Source: CAD feature listing. Evaluate the final solid. Frame: model axes, mm. Give positions to 0.01 mm unless a question says otherwise; leave off trailing zeros. Write each loop counter-clockwise with the first axis right and the second up, starting at its lowest first coordinate (ties: lowest second). Pieces come first, ordered by that corner, then holes. Notation, with made-up numbers: (78, 0) -> (90, 0) arc R28 ccw to (90, 30) -> close; hole circle Ø10 at (31, -36). An arc over 180 degrees is marked (long way). Write item = value, one per line.
from build123d import *

# Parameters (mm, degrees)
EXTRUDE_1_4_DEPTH = 3.175
SKETCH4_R         = 2
M4_DRILL_DEPTH    = 8
SKETCH5_R         = 2
M4_DRILL2_DEPTH   = 8
SKETCH6_R         = 2.25
M4_THROUGH_DEPTH  = 6.35
SKETCH8_R         = 2.25
M4_THROUGH2_DEPTH = 10


with BuildPart() as part:
    # Sketch1 → 1/4 (new, symmetric)
    with BuildSketch(Plane.XY):
        Polygon((-20, 45), (20, 45), (30, 10), (30, -45), (-30, -45), (-30, 10), align=None)
    extrude(amount=EXTRUDE_1_4_DEPTH, both=True)

    # Sketch4 → M4_DRILL (cut)
    with BuildSketch(Plane(origin=(0, 45, 0), x_dir=(1, 0, 0), z_dir=(0, 1, 0))):
        with Locations(Location((-12, 0, 0), (0, 0, 180))):
            Circle(SKETCH4_R)
        with Locations((12, 0)):
            Circle(SKETCH4_R)
    extrude(amount=-M4_DRILL_DEPTH, mode=Mode.SUBTRACT)

    # Sketch5 → M4_DRILL2 (cut)
    with BuildSketch(Plane(origin=(0, -45, 0), x_dir=(-1, 0, 0), z_dir=(0, -1, 0))):
        with Locations(Location((-20, 0, 0), (0, 0, 180))):
            Circle(SKETCH5_R)
        with Locations((20, 0)):
            Circle(SKETCH5_R)
        with Locations(Location((0, 0, 0), (0, 0, 180))):
            Circle(SKETCH5_R)
    extrude(amount=-M4_DRILL2_DEPTH, mode=Mode.SUBTRACT)

    # Sketch6 → M4_through (cut)
    with BuildSketch(Plane.XY.offset(3.175)):
        with Locations((-25.2375, -31)):
            Circle(SKETCH6_R)
        with Locations((25.2375, -31)):
            Circle(SKETCH6_R)
        with Locations((-15.2375, 31)):
            Circle(SKETCH6_R)
        with Locations((15.2375, 31)):
            Circle(SKETCH6_R)
    extrude(amount=-M4_THROUGH_DEPTH, mode=Mode.SUBTRACT)

    # Sketch8 → M4_through2 (cut)
    with BuildSketch(Plane(origin=(0, 0, -3.175), x_dir=(-1, 0, 0), z_dir=(0, 0, -1))):
        with Locations((0, 16.5)):
            Circle(SKETCH8_R)
        with Locations((16.5, 0)):
            Circle(SKETCH8_R)
        with Locations((0, -16.5)):
            Circle(SKETCH8_R)
        with Locations((-16.5, 0)):
            Circle(SKETCH8_R)
    extrude(amount=-M4_THROUGH2_DEPTH, mode=Mode.SUBTRACT)


solid = part.part
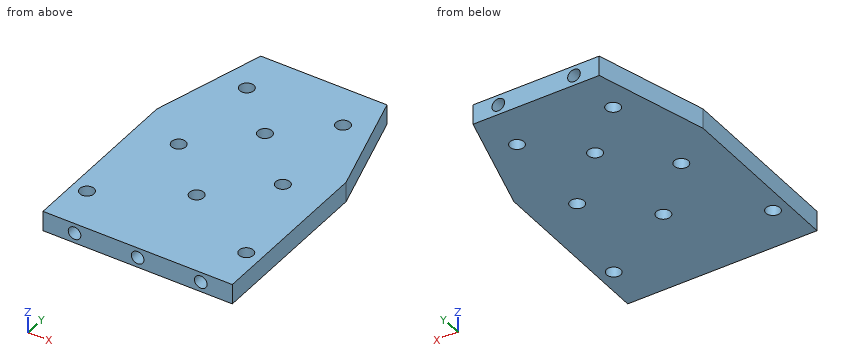
1) Material intervals for L1, parallel to Y at x = -16, z = 0.75; L2, parallel to X at y = -1.5, z = -1.75; L3, parallel to Y at x = -0.5, z = 1, sorted ascending.
Computed:
L1 = -45 to -2.19, 2.19 to 28.88, 33.12 to 45
L2 = -30 to -18.18, -14.82 to 14.82, 18.18 to 30
L3 = -37 to -18.69, -14.31 to 14.31, 18.69 to 45
2) Cut plane A-A (y = -16.5). Return the cut outline in (x, z) (3 decimals), then the cut area to 3 significant figures.
Computed:
outline = (-30, -3.175) -> (-2.25, -3.175) -> (-2.25, 3.175) -> (-30, 3.175) -> close; (2.25, -3.175) -> (30, -3.175) -> (30, 3.175) -> (2.25, 3.175) -> close
area = 352 mm²
3) Cut plane D-D (y = -32). Return the cut outline in (x, z) (3 decimals), then the cut area to 3 significant figures.
Computed:
outline = (-30, -3.175) -> (-27.253, -3.175) -> (-27.253, 3.175) -> (-30, 3.175) -> close; (-23.222, -3.175) -> (23.222, -3.175) -> (23.222, 3.175) -> (-23.222, 3.175) -> close; (27.253, -3.175) -> (30, -3.175) -> (30, 3.175) -> (27.253, 3.175) -> close
area = 330 mm²
4) Cut plane B-B (x = 0). Return the cut outline in (y, z) (3 decimals).
Computed:
outline = (-45, -3.175) -> (-18.75, -3.175) -> (-18.75, 3.175) -> (-45, 3.175) -> (-45, 2) -> (-37, 2) -> (-37, -2) -> (-45, -2) -> close; (-14.25, -3.175) -> (14.25, -3.175) -> (14.25, 3.175) -> (-14.25, 3.175) -> close; (18.75, -3.175) -> (45, -3.175) -> (45, 3.175) -> (18.75, 3.175) -> close
5) Contact query for flat-ended pins moving along their axis: pin 1 (3.5 mm diameter, centred on x = 0, z = 0, fed in from -Y); pin 2 (3 mm diameter, centred on x = 12, z = 0, fed in from +Y). Output: stop coordinate, or through.
Computed:
pin_1 = -37
pin_2 = 37
6) Cut plane C-C (z = 0). State how many separate pieces and enclosed holes the cut face has, then the cut area to 3 significant figures.
Computed:
separate_pieces = 1
enclosed_holes = 8
area = 4,760 mm²
